from build123d import *

# Parameters (mm, degrees)
SKETCH1_R           = 6
BOSS_EXTRUDE1_DEPTH = 2
SKETCH2_W           = 0.509324766
SKETCH2_H           = 0.66747415
CUT_EXTRUDE3_DEPTH  = 2
SKETCH3_R           = 1.5
CUT_EXTRUDE4_DEPTH  = 2


with BuildPart() as part:
    # Sketch1 → Boss-Extrude1 (new body)
    with BuildSketch(Plane.XY):
        Circle(SKETCH1_R)
    extrude(amount=BOSS_EXTRUDE1_DEPTH)

    # Sketch2 → Cut-Extrude3 (cut)
    with BuildSketch(Plane.XY.offset(2)):
        with Locations((0, 5.833737075)):
            Rectangle(SKETCH2_W, SKETCH2_H)
        Polygon((1.232632775, 5.366141013), (1.351814887, 6.022888578), (0.850675179, 6.113832027), (0.731493067, 5.457084462), align=None)
        Polygon((2.170985336, 5.059809838), (2.405518948, 5.684722413), (1.928671341, 5.863686313), (1.694137729, 5.238773739), align=None)
        Polygon((3.039560641, 4.590852212), (3.38190765, 5.163844591), (2.944678419, 5.425076896), (2.60233141, 4.852084517), align=None)
        Polygon((3.810441967, 3.974340819), (4.249599059, 4.476996555), (3.86604111, 4.812101043), (3.426884018, 4.309445307), align=None)
        Polygon((4.458852552, 3.230090842), (4.980704856, 3.646254167), (4.663146059, 4.044460304), (4.141293755, 3.628296979), align=None)
        Polygon((4.963951948, 2.382023087), (5.551726702, 2.698318169), (5.310373656, 3.146827283), (4.722598902, 2.8305322), align=None)
        Polygon((5.309505844, 1.45739515), (5.944311483, 1.663656006), (5.786921475, 2.148052644), (5.152115835, 1.941791788), align=None)
        Polygon((5.484407853, 0.485925334), (6.145841203, 0.575522569), (6.077472876, 1.080237825), (5.416039526, 0.99064059), align=None)
        Polygon((5.483036481, -0.501162522), (6.149838529, -0.531108637), (6.172689298, -0.022296726), (5.505887251, 0.007649388), align=None)
        Polygon((5.305435806, -1.472142602), (5.956174985, -1.620669574), (6.069510408, -1.124114642), (5.418771228, -0.975587671), align=None)
        Polygon((4.957314058, -2.395806808), (5.571075076, -2.658140857), (5.771252458, -2.189802589), (5.15749144, -1.92746854), align=None)
        Polygon((4.449860157, -3.242467812), (5.00691623, -3.610177306), (5.287501707, -3.185108478), (4.730445634, -2.817398984), align=None)
        Polygon((3.79938409, -3.984913232), (4.281830977, -4.446179686), (4.633806299, -4.078042361), (4.151359412, -3.616775907), align=None)
        Polygon((3.026792692, -4.599280262), (3.419124153, -5.139278193), (3.831176545, -4.839904606), (3.438845083, -4.299906676), align=None)
        Polygon((2.156917686, -5.065822641), (2.446523866, -5.66719607), (2.905409624, -5.446208335), (2.615803444, -4.844834906), align=None)
        Polygon((1.217717571, -5.369545311), (1.395290288, -6.012965602), (1.886260447, -5.877466447), (1.70868773, -5.234046157), align=None)
        Polygon((0.239379012, -5.500686377), (0.299210933, -6.165473472), (0.806485308, -6.119817952), (0.746653386, -5.455030857), align=None)
        Polygon((-0.746653386, -5.455030857), (-0.806485308, -6.119817952), (-0.299210933, -6.165473472), (-0.239379012, -5.500686377), align=None)
        Polygon((-1.70868773, -5.234046157), (-1.886260447, -5.877466447), (-1.395290288, -6.012965602), (-1.217717571, -5.369545311), align=None)
        Polygon((-2.615803444, -4.844834906), (-2.905409624, -5.446208335), (-2.446523866, -5.667196069), (-2.156917686, -5.065822641), align=None)
        Polygon((-3.438845083, -4.299906676), (-3.831176545, -4.839904606), (-3.419124153, -5.139278193), (-3.026792692, -4.599280262), align=None)
        Polygon((-4.151359412, -3.616775907), (-4.633806299, -4.078042361), (-4.281830977, -4.446179686), (-3.79938409, -3.984913232), align=None)
        Polygon((-4.730445634, -2.817398984), (-5.287501707, -3.185108478), (-5.00691623, -3.610177306), (-4.449860157, -3.242467812), align=None)
        Polygon((-5.15749144, -1.92746854), (-5.771252458, -2.189802589), (-5.571075076, -2.658140857), (-4.957314058, -2.395806808), align=None)
        Polygon((-5.418771228, -0.975587671), (-6.069510408, -1.124114642), (-5.956174985, -1.620669574), (-5.305435806, -1.472142602), align=None)
        Polygon((-5.505887251, 0.007649388), (-6.172689298, -0.022296726), (-6.149838529, -0.531108637), (-5.483036481, -0.501162522), align=None)
        Polygon((-5.416039526, 0.99064059), (-6.077472876, 1.080237825), (-6.145841203, 0.575522569), (-5.484407853, 0.485925334), align=None)
        Polygon((-5.152115835, 1.941791788), (-5.786921475, 2.148052644), (-5.944311483, 1.663656006), (-5.309505844, 1.45739515), align=None)
        Polygon((-4.722598902, 2.8305322), (-5.310373656, 3.146827283), (-5.551726702, 2.698318169), (-4.963951948, 2.382023087), align=None)
        Polygon((-4.141293755, 3.628296979), (-4.663146059, 4.044460304), (-4.980704856, 3.646254167), (-4.458852552, 3.230090842), align=None)
        Polygon((-3.426884018, 4.309445307), (-3.86604111, 4.812101043), (-4.249599059, 4.476996555), (-3.810441967, 3.974340819), align=None)
        Polygon((-2.60233141, 4.852084517), (-2.944678419, 5.425076896), (-3.38190765, 5.163844591), (-3.039560641, 4.590852212), align=None)
        Polygon((-1.694137729, 5.238773739), (-1.928671341, 5.863686313), (-2.405518948, 5.684722413), (-2.170985336, 5.059809838), align=None)
        Polygon((-0.731493067, 5.457084462), (-0.850675179, 6.113832027), (-1.351814887, 6.022888578), (-1.232632775, 5.366141013), align=None)
    extrude(amount=-CUT_EXTRUDE3_DEPTH, mode=Mode.SUBTRACT)

    # Sketch3 → Cut-Extrude4 (cut)
    with BuildSketch(Plane.XY.offset(2)):
        Circle(SKETCH3_R)
    extrude(amount=-CUT_EXTRUDE4_DEPTH, mode=Mode.SUBTRACT)


solid = part.part
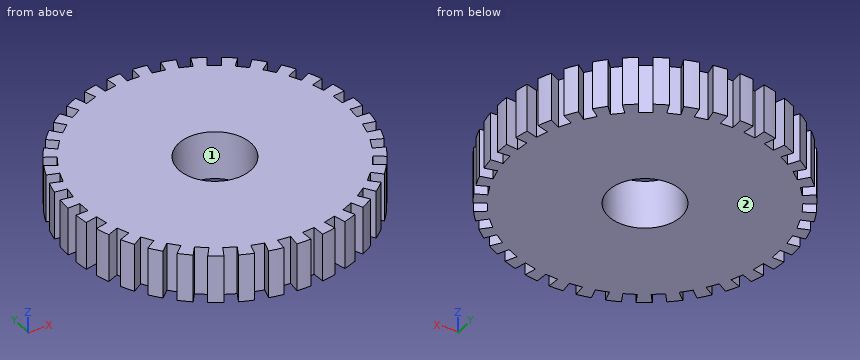
Could you check a few things on this model? Use its own coordinates, in mm. Face numbers are marked on the shaded views. Give positions to 0.01 mm unless a question says otherwise; leave off trailing zeros. Order: outer loops, then holes, each group sorted by start corner. A loop starts at its lowest first (then second) coordinate and runs counter-clockwise, first axis right, second up. Notation, with made-up numbers: M 14,15 L 32,15 A22 cw 32,49 Z; hole C 84.5,-23.5 d9. An arc over 180 degrees is marked long. One line per question, with ' | ' between items.
1. If I drill on line 1 (Y direction, x = 0, z = 1.25); line 2 (X direction, y = -4.5, z = 1.45); line 3 (X direction, y = -2, z = 1.15), over which ranges is the centre line in solid material (lowest first)?
Results:
line 1: -6 to -1.5, 1.5 to 5.5 | line 2: -3.97 to -3.58, -3.16 to 3.16, 3.58 to 3.97 | line 3: -5.66 to -5.33, -5.13 to 5.13, 5.33 to 5.66
2. We'd pull the mould along X, two halves only. Please class the marked faces 1 and 2: +X half, -X half, draft (parallel to the pull), parting line (faces both ways), or undercut.
Results:
face 1: undercut | face 2: draft
3. I want a section at A-A (x = 0). List the corners of the cut face in (y, z) for me.
Results:
outline: M -6,0 L -1.5,0 L -1.5,2 L -6,2 Z; M 1.5,0 L 5.5,0 L 5.5,2 L 1.5,2 Z
